Verification items for the finished model (mm, model axes). A direction names the side the tool comes from. Round coordinates to 2 decimals unless told otherwise and drop trailing zeros. Loops run counter-clockwise (first coordinate to the right, second up) from the corner with the lowest first, then second, coordinate; pieces in that order, holes last. Notation, with made-up numbers: M 22.5,-40 L 36.5,-40 A16 ccw 36.5,-11 Z; hole C 55,-1.5 d10. An arc over 180 degrees is marked long. Write item = value, one per line. Start each with the question number.
from build123d import *

# Parameters (mm, degrees)
F0_R     = 28.575
F1_DEPTH = 9.525
F2_R     = 23.8125
F3_DEPTH = 2.54
F4_R     = 19.773545
F5_DEPTH = 6.35


with BuildPart() as f1:
    # F0 (on Top) → F1 (new body)
    with BuildSketch(Plane.XY):
        Circle(F0_R)
    extrude(amount=F1_DEPTH)

    # F2 (on face) → F3 (cut)
    with BuildSketch(Plane(origin=(0, 0, 0), x_dir=(1, 0, 0), z_dir=(0, 0, -1))):
        Circle(F2_R)
    extrude(amount=-F3_DEPTH, mode=Mode.SUBTRACT)

    # F4 (on face) → F5 (cut)
    with BuildSketch(Plane(origin=(0, 0, 2.54), x_dir=(1, 0, 0), z_dir=(0, 0, -1))):
        Circle(F4_R)
    extrude(amount=-F5_DEPTH, mode=Mode.SUBTRACT)


solid = f1.part
1. Section check C-C, the plane z = 3.25. Enter the section's corners in (x, y) (3 decimals).
2. Section check A-A, the plane y = 0. Enter the section's corners in (x, z) (1 decimal), and give its area (3 significant figures).
3. Mould release check, pull along Y, two halves, no side actions. Record for faces 1 (the flat face through (3, -20, 2.54)), 2 (the cylindrical face through (-28.547, 1.256, 4.696)), 3 (the flat face through (-6.5, 23.4, 0)): pulls with the +Y half, pulls with the -Y half, needs draft (parallel to the pull), parting line crosses it, or undercut.
4. Section check D-D, the plane y = -21. Enter the section's corners in (x, z) (3 decimals).
5. Gauge pin test, flat ends, axial feed: P1, Ø1, axis at y = 2, z = 8, coming from the -X side; P2, Ø12, axis at x = 8.5, y = 8.5, coming from the -Z side; P3, Ø1.5, axis at y = -1, z = 3, coming from the -X side. Record the tip position at first contact, or that the pin passes through.
6. Thickness scan on line 1 (Y direction, x = 0, z = 5) (3 decimals); line 2 (Y direction, x = 0, z = 0.85) (1 decimal); line 3 (X direction, y = 14.5, z = 8.5). Record the ranges inside material, lowest first.
7. Tool access check on faces 4 (the cylindrical face through (-2.6, -19.6, 5.7)), 5 (the flat face through (0, 0, 9.525)). Record the directions out of +Z, -Z, +X, -X, +Y, -Y that give a thin tool (end or side, any length) a straight path to the whole face; none if there is none.
Computed values:
q1.outline = C 0,0 d57.15; hole C 0,0 d39.547
q2.outline = M -28.6,0 L -23.8,0 L -23.8,2.5 L -19.8,2.5 L -19.8,8.9 L 19.8,8.9 L 19.8,2.5 L 23.8,2.5 L 23.8,0 L 28.6,0 L 28.6,9.5 L -28.6,9.5 Z
q2.area = 172 mm2
q3.face_1 = undercut
q3.face_2 = parting line crosses it
q3.face_3 = needs draft
q4.outline = M -19.379,0 L -11.227,0 L -11.227,2.54 L 11.227,2.54 L 11.227,0 L 19.379,0 L 19.379,9.525 L -19.379,9.525 Z
q5.P1 = -28.54
q5.P2 = 8.89
q5.P3 = -28.57
q6.line_1 = -28.575 to -19.774, 19.774 to 28.575
q6.line_2 = -28.6 to -23.8, 23.8 to 28.6
q6.line_3 = -24.62 to -13.44, 13.44 to 24.62
q7.face_4 = -Z
q7.face_5 = +Z, +X, -X, +Y, -Y
